Work out the finished part from the listing and answer in its coordinate system (mm). Face numbers are marked on the shaded views. A direction names the side the tool comes from. Give positions to 0.01 mm unless a question says otherwise; leave off trailing zeros. Write each loop counter-clockwise with the first axis right and the second up, starting at its lowest first coordinate (ties: lowest second). Pieces come first, ordered by that corner, then holes.
1) Find section B-B (x = 65). Determine the outline of the cut face in (y, z), plus the area to 3 significant figures.
2) Given pin 1 Ø24 at (x, y) = (85, -15) entering from -Z; pin 2 Ø4.5 at (y, z) = (6.5, -7.5) entering from +X; pin 3 Ø24 at (y, z) = (-12.5, -12.5) entering from -X; pin 4 Ø8 at (x, y) = (-53, -6) entering from +Z, each flat-ended and moving along its own axis, determine where each tip first touches the part or whether it passes through.
3) Find section A-A (z = 25). Determine the outline of the cut face in (x, y), plus the area to 3 significant figures.
4) Find section C-C (y = 5.5). Determine the outline of the cut face in (x, z), plus the area to 3 significant figures.
5) Find section D-D (x = 84). Determine the outline of the cut face in (y, z).
6) A tool of negligible diameter and unlimited length cuts with its end or side. For the marked faces 4, 5 and 6, from which of +Z, -Z, +X, -X, +Y, -Y can it reach the whole face along a straight path? Write none if from no direction.
7) Straight lines are drawn through the part: probe 1 along Y at (x, z) = (91.5, 21); probe 2 along Y at (x, z) = (0.5, 49.5); probe 3 along X at (y, z) = (11, -8). For each, find the intervals that lie inside material, in ascending order.
8) Determine the mould class of the marked faces 1, 2 and 3 for opening direction X: pulls with the +X half, pulls with the -X half, needs draft (parallel to the pull), parting line crosses it, or undercut.
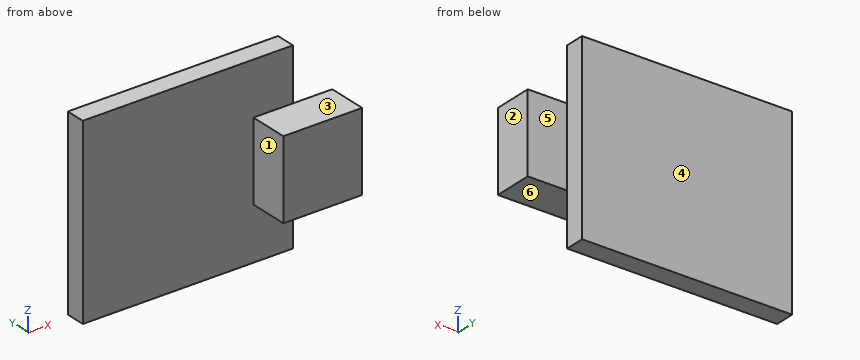
```python
from build123d import *

# Parameters (mm, degrees)
SKETCH_1_W      = 160
SKETCH_1_H      = 140
EXTRUDE_1_DEPTH = 15
SKETCH_3_W      = 60
SKETCH_3_H      = 60
EXTRUDE_2_DEPTH = 30


with BuildPart() as part:
    # 草图1 → 凸台-拉伸1 (new body)
    with BuildSketch(Plane(origin=(0, 0, 0), x_dir=(1, 0, 0), z_dir=(0, 1, 0))):
        Rectangle(SKETCH_1_W, SKETCH_1_H)
    extrude(amount=EXTRUDE_1_DEPTH)

    # 草图3 → 凸台-拉伸2 (add)
    with BuildSketch(Plane.XZ):
        with Locations((80, 0)):
            Rectangle(SKETCH_3_W, SKETCH_3_H)
    extrude(amount=EXTRUDE_2_DEPTH)


solid = part.part
```
Results:
1. outline: (-30, -30) - (0, -30) - (0, -70) - (15, -70) - (15, 70) - (0, 70) - (0, 30) - (-30, 30) - close
1. area: 3,900 mm2
2. pin 1: stops at z = -30
2. pin 2: stops at x = 80
2. pin 3: stops at x = 50
2. pin 4: passes through
3. outline: (-80, 0) - (50, 0) - (50, -30) - (110, -30) - (110, 0) - (80, 0) - (80, 15) - (-80, 15) - close
3. area: 4,200 mm2
4. outline: (-80, -70) - (80, -70) - (80, 70) - (-80, 70) - close
4. area: 22,400 mm2
5. outline: (-30, -30) - (0, -30) - (0, 30) - (-30, 30) - close
6. face 4: +Z, -Z, +X, -X, +Y
6. face 5: +Z, -Z, +X, +Y
6. face 6: -Z, +X, -X, -Y
7. probe 1: y = -30 to 0
7. probe 2: y = 0 to 15
7. probe 3: x = -80 to 80
8. face 1: pulls with the -X half
8. face 2: pulls with the +X half
8. face 3: needs draft
